from build123d import *

# Parameters (mm, degrees)
SKETCH1_R           = 2.5
BOSS_EXTRUDE1_DEPTH = 3
CUT_EXTRUDE1_DEPTH  = 1.5
CUT_EXTRUDE2_START  = 1.5
SKETCH5_R           = 2
CUT_EXTRUDE2_DEPTH  = 0.4
SKETCH7_R           = 1.5
BOSS_EXTRUDE2_DEPTH = 6
FILLET1_R           = 0.3
FILLET2_R           = 0.3


with BuildPart() as part:
    # Sketch1 → Boss-Extrude1 (new body)
    with BuildSketch(Plane(origin=(0, 0, 0), x_dir=(1, 0, 0), z_dir=(0, 1, 0))):
        with Locations(Location((0, 0, 0), (0, 0, 270))):
            Circle(SKETCH1_R)
    extrude(amount=BOSS_EXTRUDE1_DEPTH)

    # Sketch2 → Cut-Extrude1 (cut)
    with BuildSketch(Plane(origin=(0, 3, 0), x_dir=(1, 0, 0), z_dir=(0, 1, 0))):
        Polygon((2, 0), (1, 1.732050808), (-1, 1.732050808), (-2, 0), (-1, -1.732050808), (1, -1.732050808), align=None)
    extrude(amount=-CUT_EXTRUDE1_DEPTH, mode=Mode.SUBTRACT)

    # Sketch5 → Cut-Extrude2 (cut)
    with BuildSketch(Plane(origin=(0, 1.5, 0), x_dir=(1, 0, 0), z_dir=(0, 1, 0)).offset(CUT_EXTRUDE2_START)):
        with Locations(Location((0, 0, 0), (0, 0, 270))):
            Circle(SKETCH5_R)
    extrude(amount=-CUT_EXTRUDE2_DEPTH, mode=Mode.SUBTRACT)

    # Cut-Extrude3 cone 1 section (through the dimple's axis) → Cut-Extrude3 (revolve, cut)
    with BuildSketch(Plane(origin=(0, 1.5, 0), x_dir=(0, 0, 1), z_dir=(1, 0, 0))):
        Polygon((0, 0), (2, 0), (0, 0.498656006), align=None)
    revolve(axis=Axis((0, 1.5, 0), (0, -1, 0)), mode=Mode.SUBTRACT)

    # Sketch7 → Boss-Extrude2 (add)
    with BuildSketch(Plane.XZ):
        with Locations(Location((0, 0, 0), (0, 0, 270))):
            Circle(SKETCH7_R)
    extrude(amount=BOSS_EXTRUDE2_DEPTH)

    # Fillet1
    fillet1_edges = [part.edges().sort_by_distance(p)[0] for p in [
        (0, 0, -2.5),
        (0, 3, -2.5),
    ]]
    fillet(fillet1_edges, radius=FILLET1_R)

    # Fillet2
    fillet2_edges = [part.edges().sort_by_distance(p)[0] for p in [
        (0, -6, 1.5),
    ]]
    fillet(fillet2_edges, radius=FILLET2_R)


solid = part.part
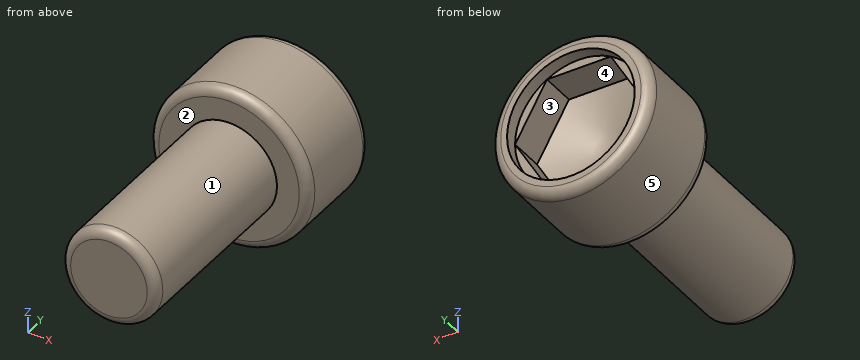
Check sheet for the modelled part. Datum: model origin and axes. Units: mm. Face numbers are marked on the shaded views. A direction names the side the tool comes from. Round coordinates to 2 decimals unless told otherwise and drop trailing zeros. Order: outer loops, then holes, each group sorted by start corner. A loop starts at its lowest first (then second) coordinate and runs counter-clockwise, first axis right, second up.
(1) Cross-section at C-C, the plane y = -4.75. Enter the section's corners in (x, z).
(2) Cross-section at A-A, the plane y = 2. Enter the section's corners in (x, z), and give its area (3 significant figures).
(3) Go/stop test with flat-tipped pins: P1, Ø2, axis at y = -4.5, z = -2, coming from the -X side; P2, Ø1.5, axis at y = 0.5, z = -1, coming from the +X side; P3, Ø0.5, axis at x = -1.5, z = -1, coming from the -Y side. Record where each tip stops, or that it passes through.
(4) Access from +Z, -Z, +X, -X, +Y, -Y to the whole of each face (thin tool, end or side, straight path). Record for the marked faces 4 and 5.
(5) Cross-section at B-B, the plane y = 0.5. Enter the section's corners in (x, z), and give its area (3 significant figures).
(6) Scan lines: probe 1 along Y at (x, z) = (-0.75, 1.9); probe 2 along X at (y, z) = (2.8, 0); probe 3 along X at (y, z) = (2.9, 0). Record each from-to range of solid material in increasing order.
(7) Draft check along Z on the marked faces 1, 2 and 3. Enter one of: pulls with the +Z half, pulls with the -Z half, needs draft (parallel to the pull), parting line crosses it, or undercut.
Check sheet entries:
1. outline: circle Ø3 at (0, 0)
2. outline: circle Ø5 at (0, 0); hole (-2, 0) - (-1, -1.73) - (1, -1.73) - (2, 0) - (1, 1.73) - (-1, 1.73) - close
2. area: 9.24 mm2
3. P1: stops at x = -1.12
3. P2: stops at x = 2.49
3. P3: stops at y = 0
4. face 4: +Y
4. face 5: +Y, -Y
5. outline: circle Ø5 at (0, 0)
5. area: 19.6 mm2
6. probe 1: y = 0 to 3
6. probe 2: x = -2.48 to -2, 2 to 2.48
6. probe 3: x = -2.42 to -2, 2 to 2.42
7. face 1: parting line crosses it
7. face 2: needs draft
7. face 3: undercut
